Could you check a few things on this model? Use its own coordinates, in mm. A direction names the side the tool comes from. Coordinates: 2 decimals unless noted, no trailing zeros. One line per item, written item: value. Start each with the question number.
(1) If we section it at A-A on y = 2.6: Count the separate pieces of the cut face and the enclosed holes in it, then the cut area to 3 significant figures.
(2) On a 3-axis mill with a long thin cutter (end or side, diameter ignored), from which of +Z, -Z, +X, -X, +Y, -Y can I reach the whole of each face in a straight line? I mean faces 1 (the face through (73.152, 3, 8)), 2 (the face through (-3, 3, 19.05)), 3 (the face through (69.9, 3, -3)). Say none if no direction works.
(3) If I drill on line 1 along Z through (x, y) = (13, 1.85); line 2 along Z through (x, y) = (5.5, 3); line 3 along X through (y, z) = (5.65, 4.5), over which ranges is the centre line in solid material (lowest first)? Write a range as from..to.
(4) I'm going to push flat-ended pins straight in: P1, Ø1, axis at x = 53.5, y = 2, coming from the -Z side; P2, Ø1, axis at x = 53, y = 3.5, coming from the +Z side; P3, Ø1.5, axis at y = 5, z = 16.5, coming from the +X side. Where does each tip first touch, or does it pass through?
(5) If we mould it in two halves opening along X, with no side actions, what happens to faces 4 (the face through (53.848, 3, 8)), 5 (the face through (12, 3, 7.772)), 6 (the face through (13.608, 3, 10)), 7 (the face through (44.5, 3, -3))? For each: pulls with the +X half, pulls with the -X half, needs draft (parallel to the pull), parting line crosses it, or undercut.
```python
from build123d import *

# Parameters (mm, degrees)
BOSS_EXTRUDE1_DEPTH = 5.842
CUT_EXTRUDE1_DEPTH  = 123.902671239
FILLET1_R           = 1
CUT_EXTRUDE2_DEPTH  = 123.902671239
SKETCH5_R           = 2.0828
CUT_EXTRUDE3_DEPTH  = 123.902671239


with BuildPart() as part:
    # Sketch1 → Boss-Extrude1 (new body)
    with BuildSketch(Plane(origin=(0, 0, 0), x_dir=(1, 0, 0), z_dir=(0, 1, 0))):
        with BuildLine():
            Line((0, 0), (6.3, 0))
            Line((6.3, 0), (6.3, 5.842))
            Line((6.3, 5.842), (19.1, 5.842))
            Line((19.1, 5.842), (19.1, 0))
            Line((19.1, 0), (31.7, 0))
            Line((31.7, 0), (31.7, 5.842))
            Line((31.7, 5.842), (44.5, 5.842))
            Line((44.5, 5.842), (44.5, 0))
            Line((44.5, 0), (57.1, 0))
            Line((57.1, 0), (57.1, 5.842))
            Line((57.1, 5.842), (69.9, 5.842))
            Line((69.9, 5.842), (69.9, 0))
            Line((69.9, 0), (82.5, 0))
            Line((82.5, 0), (82.5, 5.842))
            Line((82.5, 5.842), (95.3, 5.842))
            Line((95.3, 5.842), (95.3, 0))
            Line((95.3, 0), (111.76, 0))
            Line((111.76, 0), (111.76, -3.175))
            add(Edge.make_bspline(
                [(3.175, -50.8), (60.036806346, -32.771807959), (111.76, -3.175)],
                knots=[0, 0, 0, 1, 1, 1], degree=2))
            Line((3.175, -50.8), (0, -50.8))
            Line((0, -50.8), (0, -31.75))
            Line((0, -31.75), (-5.842, -31.75))
            Line((-5.842, -31.75), (-5.842, -19.05))
            Line((-5.842, -19.05), (0, -19.05))
            Line((0, -19.05), (0, 0))
        make_face()
    extrude(amount=BOSS_EXTRUDE1_DEPTH)

    # Sketch3 → Cut-Extrude1 (cut, through all)
    with BuildSketch(Plane(origin=(0, 5.842, 0), x_dir=(1, 0, 0), z_dir=(0, 1, 0))):
        with BuildLine():
            Line((11.056499064, -19.28001312), (29.457386054, -14.349510311))
            ThreePointArc((29.457386054, -14.349510311), (37.234515988, -18.839638371), (32.744387927, -26.616768304))
            Line((32.744387927, -26.616768304), (14.343500936, -31.547271114))
            ThreePointArc((14.343500936, -31.547271114), (6.566371003, -27.057143053), (11.056499064, -19.28001312))
        make_face()
    extrude(amount=-CUT_EXTRUDE1_DEPTH, mode=Mode.SUBTRACT)

    # Fillet1
    fillet1_edges = [part.edges().sort_by_distance(p)[0] for p in [
        (3.175, 2.921, 50.8),
        (111.76, 2.921, 3.175),
    ]]
    fillet(fillet1_edges, radius=FILLET1_R)

    # Sketch4 → Cut-Extrude2 (cut, through all)
    with BuildSketch(Plane(origin=(0, 5.842, 0), x_dir=(1, 0, 0), z_dir=(0, 1, 0))):
        Polygon((49.0474, -6.35), (47.752, -6.35), (47.752, -9.525), (49.0474, -9.525), (49.0474, -13.608), (52.5526, -13.608), (52.5526, -9.525), (53.848, -9.525), (53.848, -6.35), (52.5526, -6.35), (52.5526, 0), (49.0474, 0), align=None)
        Polygon((74.4474, -6.35), (73.152, -6.35), (73.152, -9.525), (74.4474, -9.525), (74.4474, -13.608), (77.9526, -13.608), (77.9526, -9.525), (79.248, -9.525), (79.248, -6.35), (77.9526, -6.35), (77.9526, 0), (74.4474, 0), align=None)
        Polygon((9.525, -7.7724), (9.525, -6.477), (6.35, -6.477), (6.35, -7.7724), (0, -7.7724), (0, -11.2776), (6.35, -11.2776), (6.35, -12.573), (9.525, -12.573), (9.525, -11.2776), (13.607999962, -11.2776), (13.607999962, -7.7724), align=None)
        Polygon((6.35, -43.0276), (6.35, -44.323), (9.525, -44.323), (9.525, -43.0276), (13.607999962, -43.0276), (13.607999962, -39.5224), (9.525, -39.5224), (9.525, -38.227), (6.35, -38.227), (6.35, -39.5224), (0, -39.5224), (0, -43.0276), align=None)
    extrude(amount=-CUT_EXTRUDE2_DEPTH, mode=Mode.SUBTRACT)

    # Sketch5 → Cut-Extrude3 (cut, through all)
    with BuildSketch(Plane(origin=(0, 5.842, 0), x_dir=(1, 0, 0), z_dir=(0, 1, 0))):
        with Locations(Location((44.45, -28.575, 0), (0, 0, 270))):
            Circle(SKETCH5_R)
    extrude(amount=-CUT_EXTRUDE3_DEPTH, mode=Mode.SUBTRACT)


solid = part.part
```
Values:
1. separate pieces: 1
1. enclosed holes: 2
1. area: 3,110 mm2
2. face 1: +Y, -Y
2. face 2: -Z, -X, +Y, -Y
2. face 3: -Z, +Y, -Y
3. line 1: z = -5.84..7.77, 11.28..18.76, 31.76..39.52, 43.03..47.59
3. line 2: z = 0..7.77, 11.28..39.52, 43.03..50.06
3. line 3: x = 0..49.05, 52.55..74.45, 77.95..109.43
4. P1: stops at z = 0
4. P2: stops at z = 32.58
4. P3: stops at x = 88.53
5. face 4: undercut
5. face 5: needs draft
5. face 6: pulls with the -X half
5. face 7: undercut
